Read the model definition and answer for the solid it produces. Units are mm, in the model's axes. A direction names the side the tool comes from. Round coordinates to 2 decimals unless told otherwise and drop trailing zeros. Answer as CSV lines item,"result".
```python
from build123d import *

# Parameters (mm, degrees)
SKETCH1_W                 = 31.75
SKETCH1_H                 = 6.35
BOSS_EXTRUDE1_DEPTH       = 74.93
F_4_40_TAPPED_HOLE1_D     = 2.2606
F_4_40_TAPPED_HOLE1_DEPTH = 7.5946
F_4_40_TAPPED_HOLE1_TIP   = 0.679152758
F_4_40_TAPPED_HOLE2_D     = 2.2606
F_4_40_TAPPED_HOLE2_DEPTH = 7.5946
F_4_40_TAPPED_HOLE2_TIP   = 0.679152758


with BuildPart() as part:
    # Sketch1 → Boss-Extrude1 (new body)
    with BuildSketch(Plane(origin=(0, 0, 0), x_dir=(1, 0, 0), z_dir=(0, 1, 0))):
        Rectangle(SKETCH1_W, SKETCH1_H)
    extrude(amount=BOSS_EXTRUDE1_DEPTH)

    # #4-40 Tapped Hole1
    with Locations(Plane(origin=(0, 0, 0), x_dir=(-1, 0, 0), z_dir=(0, -1, 0))):
        with Locations((9.525, 0), (-9.525, 0)):
            Hole(F_4_40_TAPPED_HOLE1_D / 2, depth=F_4_40_TAPPED_HOLE1_DEPTH)
            with Locations((0, 0, -(F_4_40_TAPPED_HOLE1_DEPTH + F_4_40_TAPPED_HOLE1_TIP / 2))):  # 118° drill point
                Cone(0, F_4_40_TAPPED_HOLE1_D / 2, F_4_40_TAPPED_HOLE1_TIP, mode=Mode.SUBTRACT)

    # #4-40 Tapped Hole2
    with Locations(Plane(origin=(0, 74.93, 0), x_dir=(1, 0, 0), z_dir=(0, 1, 0))):
        with Locations((-9.525, 0), (9.525, 0)):
            Hole(F_4_40_TAPPED_HOLE2_D / 2, depth=F_4_40_TAPPED_HOLE2_DEPTH)
            with Locations((0, 0, -(F_4_40_TAPPED_HOLE2_DEPTH + F_4_40_TAPPED_HOLE2_TIP / 2))):  # 118° drill point
                Cone(0, F_4_40_TAPPED_HOLE2_D / 2, F_4_40_TAPPED_HOLE2_TIP, mode=Mode.SUBTRACT)


solid = part.part
```
Item 1: Find the intervals of material crossed by probe 1 along X at (y, z) = (8, 0.25) (3 decimals); probe 2 along Z at (x, y) = (10.5, 72.5) (3 decimals); probe 3 along Y at (x, z) = (-9, -0.75), in increasing order. Write a range as [from, to].
Ans:
probe 1,"[-15.875, -9.906], [-9.144, 9.144], [9.906, 15.875]"
probe 2,"[-3.175, -0.572], [0.572, 3.175]"
probe 3,"[7.72, 67.21]"
Item 2: A tool of negligible diameter and unlimited length cuts with its end or side. For faces 5 (the face through (10.57, 3.85, 0.43)), 6 (the face through (10.654, 71.08, -0.05)), 7 (the face through (0, 37, -3.175)), from which of +Z, -Z, +X, -X, +Y, -Y can it reach the whole face along a straight path? Write none if from no direction.
Ans:
face 5,"-Y"
face 6,"+Y"
face 7,"-Z, +X, -X, +Y, -Y"
Item 3: A flat-ended cylindrical pin translates along its axis: pin 1 (1.8 mm diameter, centred on x = 9.525, z = 0, fed in from +Y). Find the tip coordinate at first contact, or state that the pin passes through.
Ans:
pin 1,"y = 67.2"
Item 4: Determine the mould class of faces 1 (the face through (9.329, 66.774, -0.009)), 2 (the face through (-9.4, 66.8, 0.2)), 3 (the face through (0, 37, 3.175)), 4 (the face through (0, 74.93, 0)) for opening direction Z: +Z half, -Z half, draft (parallel to the pull), parting line (faces both ways), or undercut.
Ans:
face 1,"undercut"
face 2,"undercut"
face 3,"+Z half"
face 4,"draft"
